Here's how the part is built. I have some questions about the finished solid (model axes, mm). A direction names the side the tool comes from. Coordinates: 2 decimals unless noted, no trailing zeros. Order: outer loops, then holes, each group sorted by start corner. A loop starts at its lowest first (then second) coordinate and runs counter-clockwise, first axis right, second up. Notation, with made-up numbers: (86.5, 8) - (106.5, 8) arc R16 ccw to (106.5, 39) - close; hole circle Ø5 at (39, -17.5). An arc over 180 degrees is marked (long way). Answer in a Markdown table with one row per item. Add a question column.
Item 1: If I drill on line 1 along Y through (x, z) = (-0.2, -1.1); line 2 along Y through (x, z) = (-5, 1); line 3 along Y through (x, z) = (-1.75, -1.75), over which ranges is the centre line in solid material (lowest first)? Write a range as from..to.
Item 2: On a 3-axis mill with a long thin cutter (end or side, diameter ignored), from which of +Z, -Z, +X, -X, +Y, -Y can I reach the whole of each face in a straight line? I mean faces 1 (the flat face through (-2.2, -2, 0)), 2 (the flat face through (1.55, 13, 0)), 3 (the flat face through (-4.86, 10.74, -2)). Say none if no direction works.
Item 3: I want a section at B-B (z = -1). Please give me the cut outline in (x, y).
Item 4: Thinking about a two-plate mould opening in X: for faces 4 (the cylindrical face through (-0.58, 17.21, 0.03)), 5 (the cylindrical face through (-0.579, 17.718, 0.028)), 6 (the flat face through (-4.86, 10.74, 2)), which applies, +X half, -X half, draft (parallel to the pull), parting line (faces both ways), or undercut?
Item 5: Will these pins go through, and if not, where does the flat tip stop? pin 1 Ø1.2 at (x, z) = (-9.5, -1) entering from +Y; pin 2 Ø0.6 at (y, z) = (10, 0) entering from +X; pin 3 Ø1.6 at (y, z) = (-2.5, 0) entering from +X; pin 4 Ø1.5 at (y, z) = (10.5, -1) entering from +X.
Item 6: I want a section at A-A (x = -12). Please give me the cut outline in (y, z).
```python
from build123d import *

# Parameters (mm, degrees)
SKETCH_1_W        = 20
SKETCH_1_H        = 10
EXTRUDE_1_DEPTH   = 3.2
SKETCH_2_W        = 0.5
SKETCH_2_H        = 3.2
EXTRUDE_1_2_DEPTH = 4
EXTRUDE_2_DEPTH   = 2


with BuildPart() as part:
    # Эскиз1 → Extrude 1 (new, symmetric)
    with BuildSketch(Plane.XY):
        with Locations((-10, 5)):
            Rectangle(SKETCH_1_W, SKETCH_1_H)
    extrude(amount=EXTRUDE_1_DEPTH, both=True)

    # Эскиз2 → Extrude 1 2 (add)
    with BuildSketch(Plane.XZ):
        with Locations((-18.05, 0)):
            Rectangle(SKETCH_2_W, SKETCH_2_H)
        with Locations((-9.25, 0)):
            Rectangle(SKETCH_2_W, SKETCH_2_H)
        with Locations((-1.95, 0)):
            Rectangle(SKETCH_2_W, SKETCH_2_H)
    extrude(amount=EXTRUDE_1_2_DEPTH)

    # Эскиз3 → Вытянуть-Тонкостенный2 (add, symmetric)
    with BuildSketch(Plane.XY):
        with BuildLine():
            Line((-16.95, 10), (-16.95, 10.561276731))
            Line((-16.95, 10.561276731), (2.05, 10.561276731))
            Line((2.05, 10.561276731), (2.05, 15.5))
            ThreePointArc((2.05, 15.5), (-0.634058048, 17.70773495), (-2.282527654, 14.648191002))
            Line((-2.282527654, 14.648191002), (-1.819743731, 14.83748189))
            ThreePointArc((-1.819743731, 14.83748189), (-0.537600704, 17.217127184), (1.55, 15.5))
            Line((1.55, 15.5), (1.55, 11.061276731))
            Line((1.55, 11.061276731), (-17.45, 11.061276731))
            Line((-17.45, 11.061276731), (-17.45, 10))
            Line((-17.45, 10), (-16.95, 10))
        make_face()
    extrude(amount=EXTRUDE_2_DEPTH, both=True)


solid = part.part
```
Values follow:
| question | item | result |
|---|---|---|
| 1 | line 1 | y = 0..10, 10.56..11.06, 17.25..17.75 |
| 1 | line 2 | y = 0..10, 10.56..11.06 |
| 1 | line 3 | y = 0..10, 10.56..11.06, 16.31..17.13 |
| 2 | face 1 | +Z, -Z, -Y |
| 2 | face 2 | +Z, -Z |
| 2 | face 3 | -Z, +X, -X, +Y |
| 3 | outline | (-20, 0) - (-18.3, 0) - (-18.3, -4) - (-17.8, -4) - (-17.8, 0) - (-9.5, 0) - (-9.5, -4) - (-9, -4) - (-9, 0) - (-2.2, 0) - (-2.2, -4) - (-1.7, -4) - (-1.7, 0) - (0, 0) - (0, 10) - (-16.95, 10) - (-16.95, 10.56) - (2.05, 10.56) - (2.05, 15.5) arc R2.25 ccw (long way) to (-2.28, 14.65) - (-1.82, 14.84) arc R1.75 cw (long way) to (1.55, 15.5) - (1.55, 11.06) - (-17.45, 11.06) - (-17.45, 10) - (-20, 10) - close |
| 4 | face 4 | undercut |
| 4 | face 5 | parting line |
| 4 | face 6 | draft |
| 5 | pin 1 | stops at y = 11.06 |
| 5 | pin 2 | stops at x = 0 |
| 5 | pin 3 | stops at x = -1.7 |
| 5 | pin 4 | stops at x = 2.05 |
| 6 | outline | (0, -3.2) - (10, -3.2) - (10, 3.2) - (0, 3.2) - close; (10.56, -2) - (11.06, -2) - (11.06, 2) - (10.56, 2) - close |
